Input: part model. Units: mm. Frame: model coordinates. A direction names the side the tool comes from. Round coordinates to 2 decimals unless told otherwise and drop trailing zeros. Loops run counter-clockwise (first coordinate to the right, second up) from the corner with the lowest first, then second, coordinate; pieces in that order, holes last. Notation, with made-up numbers: (-24.5, 88.25) - (33.5, 88.25) arc R33 ccw to (33.5, 126.25) - close; hole circle Ø11 at (-17.75, -24). An arc over 180 degrees is marked (long way). One line per question, with ' | ' between items. Start each with the question number.
Item 1: Set-up query: faces 1 (the face through (-5, 5, 12.7)), 2 (the face through (0, 1.27, 14)). Return all of +Z, -Z, +X, -X, +Y, -Y with unobstructed straight access to the full face (end or side cutting, diameter ignored); none if empty.
Item 2: First-contact query: pin 1 (2 mm diameter, centred on y = 0.5, z = 14, fed in from +X); pin 2 (6 mm diameter, centred on y = 6, z = 8.5, fed in from -X); pin 3 (1 mm diameter, centred on x = -8, y = 5, fed in from +Z). Flat tips, straight axial feed; report the tip coordinate or a pass-through.
Item 3: Draft query along X for faces 3 (the face through (-1.38, 6.2, 6.44)), 4 (the face through (0, 0, 0)), 5 (the face through (-5.08, 0, 14)). Return one class per face: pulls with the +X half, pulls with the -X half, needs draft (parallel to the pull), parting line crosses it, or undercut.
Item 4: Section A-A, the plane z = 3.25. Return loops of the section in (x, y), plus the area to 3 significant figures.
Item 5: Material intervals for line 1 along Z through (x, y) = (4, -0.25); line 2 along Y through (x, z) = (4, 14.5); line 3 along X through (y, z) = (1, 9.25), sorted ascending.
```python
from build123d import *

# Parameters (mm, degrees)
F2_W     = 10.16
F2_H     = 2.54
F3_DEPTH = 25.4


with BuildPart() as f1:
    # F0 (on Front) → F1 (revolve)
    with BuildSketch(Plane.XZ):
        with BuildLine():
            Line((0, 15.875), (0, 0))
            Line((0, 0), (6.35, 0))
            Line((6.35, 0), (6.35, 12.7))
            Line((6.35, 12.7), (11.43, 12.7))
            ThreePointArc((11.43, 12.7), (6.055334, 15.512702), (0, 15.875))
        make_face()
    revolve(axis=Axis((0, 0, 4.292885), (0, 0, -1)))

    # F2 (on face) → F3 (cut)
    with BuildSketch(Plane(origin=(0, 0, 12.7), x_dir=(1, 0, 0), z_dir=(0, 0, -1))):
        Rectangle(F2_W, F2_H)
    extrude(amount=-F3_DEPTH, mode=Mode.SUBTRACT)


solid = f1.part
```
Return value:
1) face 1: -Z | face 2: +Z
2) pin 1: x = 11.05 | pin 2: x = -5.6 | pin 3: z = 14.37
3) face 3: parting line crosses it | face 4: needs draft | face 5: undercut
4) outline: circle Ø12.7 at (0, 0) | area: 127 mm2
5) line 1: 0 to 12.7 | line 2: -7.7 to -1.27, 1.27 to 7.7 | line 3: -6.27 to 6.27
